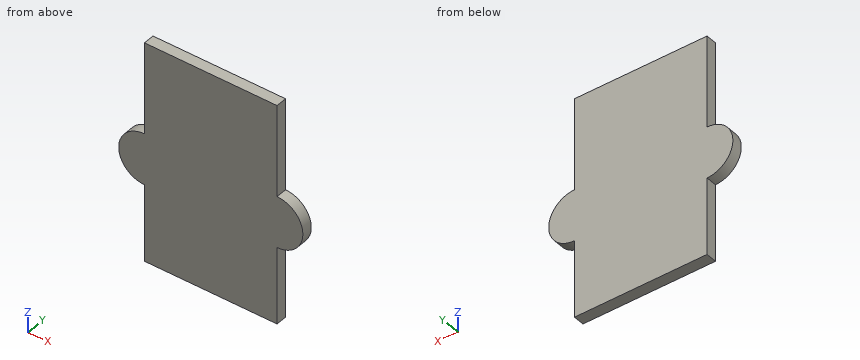
Autodesk Inventor part; units mm, degrees
ref_plane "YZ Plane" through (0, 0, 0) normal (1, 0, 0) x (0, 1, 0)
ref_plane "XZ Plane" through (0, 0, 0) normal (0, 1, 0) x (-1, 0, 0)
ref_plane "XY Plane" through (0, 0, 0) normal (0, 0, 1) x (1, 0, 0)
sketch "スケッチ1" plane through (0, 0, 0) normal (0, 1, 0) x (-1, 0, 0)
  line L0 (0, 0) -> (25, 0)
  line L1 (25, 0) -> (25, -30)
  line L2 (25, -30) -> (0, -30)
  line L3 (0, -30) -> (0, 0)
  circle A0 centre (21.5, -16) radius 3.5
  circle A1 centre (3.5, -16) radius 3.5
  line L4 (21.5, 0) -> (21.5, -30)
  line L5 (3.5, -30) -> (3.5, 0)
  point P0 (21.5, -19.5)
  point P1 (21.5, -12.5)
  point P2 (3.5, -12.5)
  point P3 (3.5, -19.5)
  dimension "d0" = 25
  dimension "d1" = 30
  dimension "d2" = 7
  dimension "d3" = 16
extrude "押し出し1" add sketch "スケッチ1" along normal blind 1.5 contours L0 L4 A0 L2 L5 A1 | A1 L5 | A1 L5 | L4 A0 | A0 L4
properties part number "type_C"
Source: CAD feature listing. Evaluate the final solid. Frame: model axes, mm. Give positions to 0.01 mm unless a question says otherwise; leave off trailing zeros. Write each loop counter-clockwise with the first axis right and the second up, starting at its lowest first coordinate (ties: lowest second). Pieces come first, ordered by that corner, then holes. Notation, with made-up numbers: M 0,2.25 L 37,2.25 A33 cw 37,39.25 Z; hole C -16,84 d8. An arc over 180 degrees is marked long. Return JSON: item names as keys, results as strings. Group by question number.
1) Pin query (flat end, axial travel): P1, Ø0.8, axis at y = 1, z = -4.5, coming from the -X side. Return the tip coordinate at first contact, or that it passes through.
2) Cut plane B-B, the plane z = -20.5. Output: boundary loops of the cut face in (x, y).
3) Cut plane A-A, the plane y = 0.7. Output: boundary loops of the cut face in (x, z), plus the area to 3 significant figures.
4) Material intervals for line 1 along X through (y, z) = (0.8, -28.5); line 2 along X through (y, z) = (0.7, -18.25); line 3 along Z through (x, y) = (-2, 0.2), sorted ascending. Write a range as [from, to].
Recorded:
{
 "1": {"P1": "stops at x = -21.5"},
 "2": {"outline": "M -21.5,0 L -3.5,0 L -3.5,1.5 L -21.5,1.5 Z"},
 "3": {"outline": "M -21.5,-30 L -3.5,-30 L -3.5,-19.5 A3.5 ccw -3.5,-12.5 L -3.5,0 L -21.5,0 L -21.5,-12.5 A3.5 ccw -21.5,-19.5 Z", "area": "578 mm²"},
 "4": {"line 1": "x = [-21.5, -3.5]", "line 2": "x = [-24.18, -0.82]", "line 3": "z = [-19.16, -12.84]"}
}
